Design review of the part built by this model. Coordinates are the model's own, in mm. Face numbers are marked on the shaded views. A direction names the side the tool comes from. Give positions to 0.01 mm unless a question says otherwise; leave off trailing zeros. Write each loop counter-clockwise with the first axis right and the second up, starting at its lowest first coordinate (ties: lowest second). Pieces come first, ordered by that corner, then holes. Notation, with made-up numbers: (12.5, -24) -> (31.5, -24) arc R22 ccw to (31.5, 15) -> close; hole circle Ø11 at (32, 14.25). An arc over 180 degrees is marked (long way). Use CSV: the item, a comma, the result in double quotes.
```python
from build123d import *

# Parameters (mm, degrees)
BASE_FLANGE1_DEPTH      = 70
CUT_EXTRUDE2_DEPTH      = 99.666559685
CUT_EXTRUDE2_DEPTH_BACK = 99.666559685
SKETCH6_R               = 22.25
CUT_EXTRUDE3_START      = -24.7
CUT_EXTRUDE3_DEPTH      = 24.7
FILLET1_R               = 10
FILLET2_R               = 5


# Read off the part's stored shape, not the designer's step: Cut-Extrude3
# Sheet-metal steps are written as plain solids
with BuildPart() as part:
    # Sketch1 → Base-Flange1 (new, symmetric)
    with BuildSketch(Plane(origin=(0, 0, 0), x_dir=(0, 0, -1), z_dir=(1, 0, 0))):
        with BuildLine():
            Line((0, 0), (-59.22, 0))
            ThreePointArc((-59.22, 0), (-63.307077195, 1.692922805), (-65, 5.78))
            Line((-65, 5.78), (-65, 18.92))
            ThreePointArc((-65, 18.92), (-63.307077195, 23.007077195), (-59.22, 24.7))
            Line((-59.22, 24.7), (0, 24.7))
            Line((0, 24.7), (0, 19.7))
            Line((0, 19.7), (-59.22, 19.7))
            ThreePointArc((-59.22, 19.7), (-59.771543289, 19.471543289), (-60, 18.92))
            Line((-60, 18.92), (-60, 5.78))
            ThreePointArc((-60, 5.78), (-59.771543289, 5.228456711), (-59.22, 5))
            Line((-59.22, 5), (0, 5))
            Line((0, 5), (0, 0))
        make_face()
    extrude(amount=BASE_FLANGE1_DEPTH, both=True)

    # Sketch6 → Cut-Extrude2 (cut, two sides: drawn at the far end of the back side and taken through both)
    with BuildSketch(Plane(origin=(0, 0, 0), x_dir=(1, 0, 0), z_dir=(0, 1, 0)).offset(-CUT_EXTRUDE2_DEPTH_BACK)):
        with Locations(Location((36, -32.7, 0), (0, 0, 270))):
            Circle(SKETCH6_R)
    extrude(amount=CUT_EXTRUDE2_DEPTH + CUT_EXTRUDE2_DEPTH_BACK, mode=Mode.SUBTRACT)

    # Cut-Extrude3 outline → Cut-Extrude3 (cut)
    with BuildSketch(Plane(origin=(0, 24.7, 0), x_dir=(1, 0, 0), z_dir=(0, 1, 0)).offset(CUT_EXTRUDE3_START)):
        with BuildLine():
            add(Edge.make_bspline(
                [(-28, -59.22), (-28.001483373, -59.059147185), (-28.006444043, -58.521225961), (-28.068654058, -57.607370733), (-28.221663959, -56.485748427), (-28.454487396, -55.377760999), (-28.76476049, -54.288987367), (-29.151253932, -53.224858787), (-29.611949694, -52.190697164), (-30.144568106, -51.191670906), (-30.746440721, -50.232773794), (-31.414560774, -49.318798758), (-32.145588265, -48.454314261), (-32.935869316, -47.643641371), (-33.781453727, -46.890832185), (-34.678114904, -46.199649575), (-35.621370941, -45.573548372), (-36.606507032, -45.015658105), (-37.628599035, -44.528767354), (-38.682538088, -44.11530981), (-39.763056142, -43.777352116), (-40.864752295, -43.516583532), (-41.982119787, -43.334307495), (-43.109573528, -43.231435098), (-44.24147801, -43.208480544), (-45.372175479, -43.265558569), (-46.496014214, -43.402383872), (-47.607376779, -43.618272541), (-48.700708096, -43.91214547), (-49.770543218, -44.282533752), (-50.81153464, -44.727586026), (-51.818479031, -45.245077726), (-52.786343244, -45.832422201), (-53.71028947, -46.486683647), (-54.585699418, -47.204591779), (-55.408197421, -47.982558178), (-56.17367222, -48.816694228), (-56.878297832, -49.702830551), (-57.518551508, -50.636537851), (-58.091235675, -51.613149051), (-58.593477749, -52.627782619), (-59.022804836, -53.675366973), (-59.376930909, -54.75066583), (-59.654608607, -55.848304374), (-59.852499172, -56.962796127), (-59.976893957, -58.088570374), (-59.992297986, -58.842856791), (-60, -59.22)],
                knots=[0, 0, 0, 0, 0.009602085, 0.032111129, 0.054620172, 0.077129216, 0.099638259, 0.122147303, 0.144656346, 0.16716539, 0.189674433, 0.212183477, 0.23469252, 0.257201564, 0.279710607, 0.302219651, 0.324728695, 0.347237738, 0.369746782, 0.392255825, 0.414764869, 0.437273912, 0.459782956, 0.482291999, 0.504801043, 0.527310086, 0.54981913, 0.572328173, 0.594837217, 0.61734626, 0.639855304, 0.662364347, 0.684873391, 0.707382434, 0.729891478, 0.752400521, 0.774909565, 0.797418608, 0.819927652, 0.842436695, 0.864945739, 0.887454782, 0.909963826, 0.932472869, 0.954981913, 0.977490956, 1, 1, 1, 1], degree=3))
            Line((-60, -59.22), (-60, -65))
            Line((-60, -65), (-28, -65))
            Line((-28, -65), (-28, -59.22))
        make_face()
        Polygon((-13.431457505, -9), (38.798801924, 0), (-70, 0), (-70, -29), align=None)
        with BuildLine():
            ThreePointArc((38.798801924, 0), (57.406545367, -6.032071037), (70, -21))
            Line((70, -21), (70, 0))
            Line((70, 0), (38.798801924, 0))
        make_face()
        Polygon((70, -65), (70, -50), (60, -59.22), (60, -65), align=None)
    extrude(amount=CUT_EXTRUDE3_DEPTH, mode=Mode.SUBTRACT)

    # Fillet1
    fillet1_edges = [part.edges().sort_by_distance(p)[0] for p in [
        (38.798801924, 22.2, 0),
        (-13.431457505, 22.2, 9),
        (70, 2.5, 21),
        (38.798801924, 2.5, 0),
        (-13.431457505, 2.5, 9),
        (70, 22.2, 21),
    ]]
    fillet(fillet1_edges, radius=FILLET1_R)

    # Fillet2
    fillet2_edges = [part.edges().sort_by_distance(p)[0] for p in [
        (-70, 22.2, 29),
        (70, 2.5, 50),
        (70, 22.2, 50),
        (-70, 2.5, 29),
    ]]
    fillet(fillet2_edges, radius=FILLET2_R)


solid = part.part
```
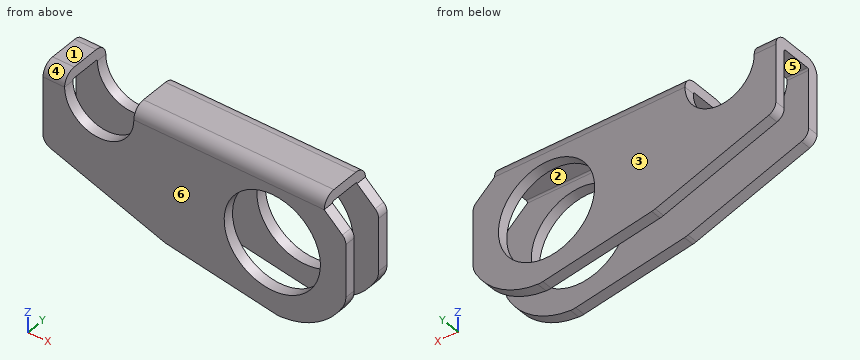
(1) Clearance check with flat-ended pins moving along their axes: pin 1 (6 mm diameter, centred on y = 15.5, z = 17, fed in from -X); pin 2 (10.5 mm diameter, centred on x = -2.5, y = 11.5, fed in from -Z); pin 3 (3 mm diameter, centred on y = 17, z = 63, fed in from +X); pin 4 (5 mm diameter, centred on x = -1, y = 19.5, fed in from +Z). State where each tip first meets the part, or that it passes through.
Established:
pin 1,"passes through"
pin 2,"stops at z = 60"
pin 3,"stops at x = 60"
pin 4,"stops at z = 65"
(2) Take a section at B-B (x = 36). Write out the cut boundary in (y, z), then the cut area to 3 significant figures.
Established:
outline,"(0, 0.48) -> (5, 0.48) -> (5, 10.45) -> (0, 10.45) -> close; (0, 54.95) -> (5, 54.95) -> (5, 59.22) arc R0.78 cw to (5.78, 60) -> (18.92, 60) arc R0.78 cw to (19.7, 59.22) -> (19.7, 54.95) -> (24.7, 54.95) -> (24.7, 59.22) arc R5.78 ccw to (18.92, 65) -> (5.78, 65) arc R5.78 ccw to (0, 59.22) -> close; (19.7, 0.48) -> (24.7, 0.48) -> (24.7, 10.45) -> (19.7, 10.45) -> close"
area,"260 mm2"
(3) Take a section at D-D (z = 5). Write out the cut boundary in (x, y).
Established:
outline,"(9.78, 0) -> (55.78, 0) -> (55.78, 5) -> (9.78, 5) -> close; (9.78, 19.7) -> (55.78, 19.7) -> (55.78, 24.7) -> (9.78, 24.7) -> close"
(4) For line 1 along Y through (x, z) = (-10.5, 49); line 2 along X through (y, z) = (2.9, 32.7); line 3 along Z through (x, y) = (50.5, 23.25), list the stretches that pass through material, from the lowest coordinate up. Write a range as [from, to].
Established:
line 1,"y = [0, 5], [19.7, 24.7]"
line 2,"x = [-70, 13.75], [58.25, 70]"
line 3,"z = [2.41, 15.82], [49.58, 63.05]"
(5) Take a section at A-A (y = 10). Write out the cut boundary in (x, z), then the cut area to 3 significant figures.
Established:
outline,"(-70, 60) -> (-60, 60) -> (-60, 65) -> (-70, 65) -> close; (-28, 60) -> (60, 60) -> (60, 65) -> (-28, 65) -> close"
area,"490 mm2"
(6) Mouldability with a two-part tool opening along Y and no side actions: class the marked faces 1, 2, 3 and 4 as +Y half, -Y half, draft (parallel to the pull), parting line (faces both ways), or undercut.
Established:
face 1,"draft"
face 2,"undercut"
face 3,"+Y half"
face 4,"-Y half"
(7) Tool access review of the marked faces 5 and 6: name each direction out of +Z, -Z, +X, -X, +Y, -Y from which nothing blocks a thin tool from reaching the whole face with its end or side.
Established:
face 5,"-Z, +X, -X"
face 6,"+Z, -Z, +X, -X, -Y"
(8) Take a section at C-C (z = 31). Write out the cut boundary in (x, y), then the cut area to 3 significant figures.
Established:
outline,"(-69.76, 0) -> (13.82, 0) -> (13.82, 5) -> (-69.76, 5) -> close; (-69.76, 19.7) -> (13.82, 19.7) -> (13.82, 24.7) -> (-69.76, 24.7) -> close; (58.18, 0) -> (70, 0) -> (70, 5) -> (58.18, 5) -> close; (58.18, 19.7) -> (70, 19.7) -> (70, 24.7) -> (58.18, 24.7) -> close"
area,"954 mm2"
